from build123d import *

# Parameters (mm, degrees)
SM_BASE_FLANGE_1_DEPTH = 6


# Sheet-metal steps are written as plain solids
with BuildPart() as part:
    # Sketch 1 → Базовая кромка1 (new body)
    with BuildSketch(Plane(origin=(0, 0, 0), x_dir=(1, 0, 0), z_dir=(0, 1, 0))):
        Polygon((0, -202.132034356), (60, -202.132034356), (252.882034356, -9.25), (252.882034356, 100), (130.626438318, 100), (130.626438318, 44), (50, 44), (50, 0), (0, 0), align=None)
    extrude(amount=-SM_BASE_FLANGE_1_DEPTH)

    # Зеркальное отражение1: part across plane


with BuildPart() as part_1:
    add(part.part)
    add(part.part.mirror(Plane(origin=(0, -6, 0), x_dir=(0, 0, 1), z_dir=(-1, 0, 0))))


solid = part_1.part
Read the model definition and answer for the solid it produces. Units are mm, in the model's axes. Round coordinates to 2 decimals unless told otherwise and drop trailing zeros. Write each loop counter-clockwise with the first axis right and the second up, starting at its lowest first coordinate (ties: lowest second). Pieces come first, ordered by that corner, then holes.
1. The part is cut by section B-B, the plane y = -3.2. Determine the outline of the cut face in (x, z), then the cut area to 3 significant figures.
2. The part is cut by section D-D, the plane z = 159. Determine the outline of the cut face in (x, y).
3. The part is cut by section C-C, the plane x = 41. Determine the outline of the cut face in (y, z), then the cut area to 3 significant figures.
4. Given pin 1 Ø3 at (x, y) = (-153.5, -1) entering from +Z, flat-ended and moving along its own axis, determine where the tip first touches the part or whether it passes through.
5. The part is cut by section A-A, the plane z = -59. Determine the outline of the cut face in (x, y).
6. Straight lines are drawn through the part: L1, parallel to X at y = -4.55, z = -0.5; L2, parallel to Z at x = 58, y = -4.1; L3, parallel to X at y = -5.6, z = -66. For each, find the intervals that lie inside material, in ascending order.
Values:
1. outline: (-252.88, -100) - (-130.63, -100) - (-130.63, -44) - (-50, -44) - (-50, 0) - (50, 0) - (50, -44) - (130.63, -44) - (130.63, -100) - (252.88, -100) - (252.88, 9.25) - (60, 202.13) - (-60, 202.13) - (-252.88, 9.25) - close
1. area: 96,600 mm2
2. outline: (-103.13, -6) - (103.13, -6) - (103.13, 0) - (-103.13, 0) - close
3. outline: (-6, 0) - (0, 0) - (0, 202.13) - (-6, 202.13) - close
3. area: 1,210 mm2
4. pin 1: stops at z = 110.13
5. outline: (-252.88, -6) - (-130.63, -6) - (-130.63, 0) - (-252.88, 0) - close; (130.63, -6) - (252.88, -6) - (252.88, 0) - (130.63, 0) - close
6. L1: x = -252.88 to -50, 50 to 252.88
6. L2: z = -44 to 202.13
6. L3: x = -252.88 to -130.63, 130.63 to 252.88
